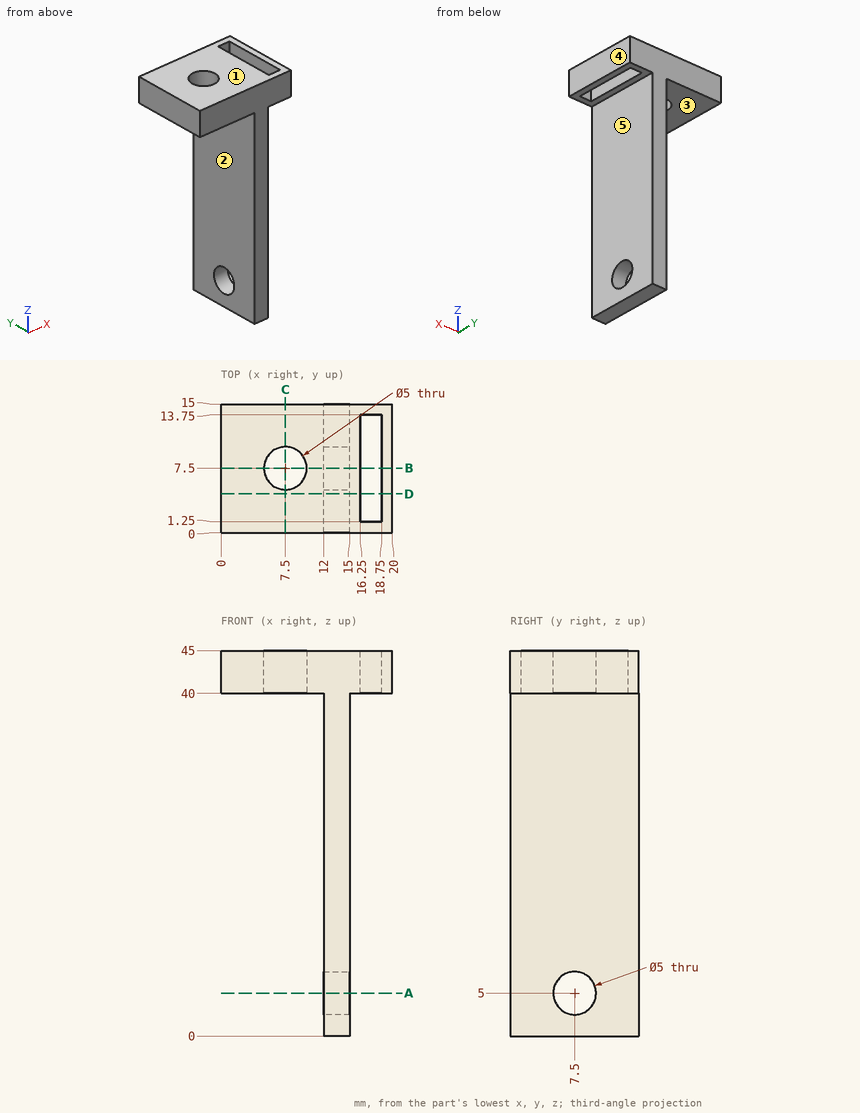
Check sheet for the drawn part. Datum: minimum x, y, z corner. Units: mm. A direction names the side the tool comes from. Give positions to 0.01 mm unless a question says otherwise; leave off trailing zeros. Order: outer loops, then holes, each group sorted by start corner. A loop starts at its lowest first (then second) coordinate and runs counter-clockwise, first axis right, second up. Notation, with made-up numbers: (-22, 28) - (-9, 28) arc R6 cw to (-9, 36) - close; hole circle Ø11 at (57.5, -29.5). An arc over 180 degrees is marked (long way). Write item = value, one per line. Start each with the question number.
1) Section check C-C (x = 7.5). Enter the section's corners in (y, z).
2) Section check D-D (y = 4.5). Enter the section's corners in (x, z).
3) Access from +Z, -Z, +X, -X, +Y, -Y to the whole of each face (thin tool, end or side, straight path). Record for the marked faces 4 and 5.
4) Section check A-A (z = 5). Enter the section's corners in (x, y), then the cut area to 3 significant figures.
5) Scan lines: L1, parallel to Y at x = 7.5, z = 42.55; L2, parallel to X at y = 11, z = 21.5; L3, parallel to Z at x = 8.25, y = 13. Record each from-to range of solid material in increasing order.
6) Draft check along Z on the marked faces 1, 2 and 3. Enter one of: released by +Z, released by -Z, zero draft, split by the parting line, or undercut.
7) Gauge pin test, flat ends, axial feed: pin 1 Ø7.5 at (y, z) = (9.5, 25) entering from +X; pin 2 Ø7.5 at (y, z) = (11, 26.5) entering from -X; pin 3 Ø2.5 at (x, y) = (18, 8) entering from -Z. Record the tip position at first contact, or that the pin passes through.
8) Section check B-B (y = 7.5). Enter the section's corners in (x, z), then the cut area to 4 significant figures.
Geometry check:
q1.outline = (0, 40) - (5, 40) - (5, 45) - (0, 45) - close; (10, 40) - (15, 40) - (15, 45) - (10, 45) - close
q2.outline = (0, 40) - (12, 40) - (12, 0) - (15, 0) - (15, 40) - (16.25, 40) - (16.25, 45) - (0, 45) - close; (18.75, 40) - (20, 40) - (20, 45) - (18.75, 45) - close
q3.face_4 = +Z, -Z, +X, +Y, -Y
q3.face_5 = -Z, +X, +Y, -Y
q4.outline = (12, 0) - (15, 0) - (15, 5) - (12, 5) - close; (12, 10) - (15, 10) - (15, 15) - (12, 15) - close
q4.area = 30.0 mm2
q5.L1 = 0 to 5, 10 to 15
q5.L2 = 12 to 15
q5.L3 = 40 to 45
q6.face_1 = released by +Z
q6.face_2 = zero draft
q6.face_3 = released by -Z
q7.pin_1 = 15
q7.pin_2 = 12
q7.pin_3 = 40
q8.outline = (0, 40) - (5, 40) - (5, 45) - (0, 45) - close; (10, 40) - (12, 40) - (12, 7.5) - (15, 7.5) - (15, 40) - (16.25, 40) - (16.25, 45) - (10, 45) - close; (12, 0) - (15, 0) - (15, 2.5) - (12, 2.5) - close; (18.75, 40) - (20, 40) - (20, 45) - (18.75, 45) - close
q8.area = 167.5 mm2
